```python
from build123d import *

# Parameters (mm, degrees)
F0_R     = 1
F0_R_2   = 12.5
F1_DEPTH = 1


with BuildPart() as f1:
    # F0 (on Top) → F1 (new body)
    with BuildSketch(Plane.XY):
        with BuildLine():
            Line((19, 25), (0, 25))
            Line((0, 25), (-19, 25))
            Line((-19, 25), (-19, 41))
            Line((-19, 41), (-25, 41))
            ThreePointArc((-25, 41), (-48.020829, 0), (-25, -41))
            Line((-25, -41), (-19, -41))
            Line((-19, -41), (-19, -25))
            Line((-19, -25), (0, -25))
            Line((0, -25), (19, -25))
            Line((19, -25), (19, -41))
            Line((19, -41), (25, -41))
            ThreePointArc((25, -41), (48.020829, 0), (25, 41))
            Line((25, 41), (19, 41))
            Line((19, 41), (19, 25))
        make_face()
        with Locations((-11, -23)):
            Circle(F0_R, mode=Mode.SUBTRACT)
        with Locations((11, -23)):
            Circle(F0_R, mode=Mode.SUBTRACT)
        with Locations((-25, 0)):
            Circle(F0_R_2, mode=Mode.SUBTRACT)
        with Locations((-11, 23)):
            Circle(F0_R, mode=Mode.SUBTRACT)
        with Locations((25, 0)):
            Circle(F0_R_2, mode=Mode.SUBTRACT)
        with Locations((11, 23)):
            Circle(F0_R, mode=Mode.SUBTRACT)
    extrude(amount=F1_DEPTH)


solid = f1.part
```
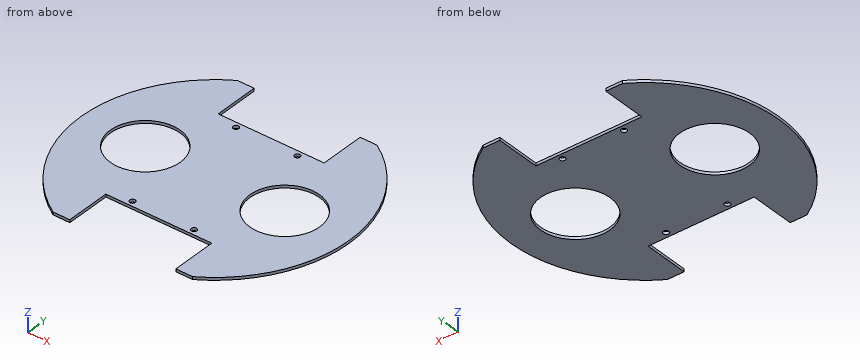
The model under review builds one solid part; all positions refer to its coordinate system, in mm. Coordinates: 2 decimals unless noted, no trailing zeros. Order: outer loops, then holes, each group sorted by start corner. A loop starts at its lowest first (then second) coordinate and runs counter-clockwise, first axis right, second up. Notation, with made-up numbers: (-9, 48) -> (33, 48) arc R29 ccw to (33, 82) -> close; hole circle Ø7 at (80.5, 20.5). An arc over 180 degrees is marked (long way). Answer in a Markdown table with one row per item. Add a question column.
Item 1: We need section B-B on y = 0. Write out the cut boundary in (x, z), plus the area to 3 significant figures.
Item 2: We need section C-C on x = -21. Write out the cut boundary in (y, z).
Item 3: We need section A-A on z = 0.15. Write out the cut boundary in (x, y), plus the area to 3 significant figures.
Item 4: To check wall thickness, follow probe 1 along Y at (x, z) = (-11, 0.4); probe 2 along X at (y, z) = (4, 0.7); probe 3 along X at (y, z) = (4.5, 0.35). State the ranges of each line that lie inside material, in increasing order.
Item 5: We need section D-D on y = -27. Write out the cut boundary in (x, z).
Item 6: Clearance check with flat-ended pins moving along their axes: pin 1 (15 mm diameter, centred on x = -25, y = 0, fed in from +Z); pin 2 (0.5 mm diameter, centred on x = -9, z = 0.5, fed in from -Y); pin 3 (0.5 mm diameter, centred on x = -6.5, z = 0.5, fed in from +Y). State where each tip first meets the part, or that it passes through.
Final values:
| question | item | result |
|---|---|---|
| 1 | outline | (-48.02, 0) -> (-37.5, 0) -> (-37.5, 1) -> (-48.02, 1) -> close; (-12.5, 0) -> (12.5, 0) -> (12.5, 1) -> (-12.5, 1) -> close; (37.5, 0) -> (48.02, 0) -> (48.02, 1) -> (37.5, 1) -> close |
| 1 | area | 46.0 mm2 |
| 2 | outline | (-41, 0) -> (-11.84, 0) -> (-11.84, 1) -> (-41, 1) -> close; (11.84, 0) -> (41, 0) -> (41, 1) -> (11.84, 1) -> close |
| 3 | outline | (-25, -41) -> (-19, -41) -> (-19, -25) -> (19, -25) -> (19, -41) -> (25, -41) arc R48.02 ccw to (25, 41) -> (19, 41) -> (19, 25) -> (-19, 25) -> (-19, 41) -> (-25, 41) arc R48.02 ccw to start; hole circle Ø25 at (-25, 0); hole circle Ø2 at (-11, -23); hole circle Ø2 at (-11, 23); hole circle Ø2 at (11, -23); hole circle Ø2 at (11, 23); hole circle Ø25 at (25, 0) |
| 3 | area | 4,560 mm2 |
| 4 | probe 1 | y = -25 to -24, -22 to 22, 24 to 25 |
| 4 | probe 2 | x = -47.85 to -36.84, -13.16 to 13.16, 36.84 to 47.85 |
| 4 | probe 3 | x = -47.81 to -36.66, -13.34 to 13.34, 36.66 to 47.81 |
| 5 | outline | (-39.71, 0) -> (-19, 0) -> (-19, 1) -> (-39.71, 1) -> close; (19, 0) -> (39.71, 0) -> (39.71, 1) -> (19, 1) -> close |
| 6 | pin 1 | passes through |
| 6 | pin 2 | stops at y = -25 |
| 6 | pin 3 | stops at y = 25 |
